Part print with two shaded views. Sizes in mm from the minimum x, y, z corner. A direction names the side the tool comes from. Round coordinates to 2 decimals unless told otherwise and drop trailing zeros. Loops run counter-clockwise (first coordinate to the right, second up) from the corner with the lowest first, then second, coordinate; pieces in that order, holes last. Notation, with made-up numbers: (66.5, 36.5) - (95.5, 36.5) arc R29 ccw to (95.5, 57.5) - close; hole circle Ø7 at (19, -8.5). An arc over 180 degrees is marked (long way). One line per question, with ' | ' between items.
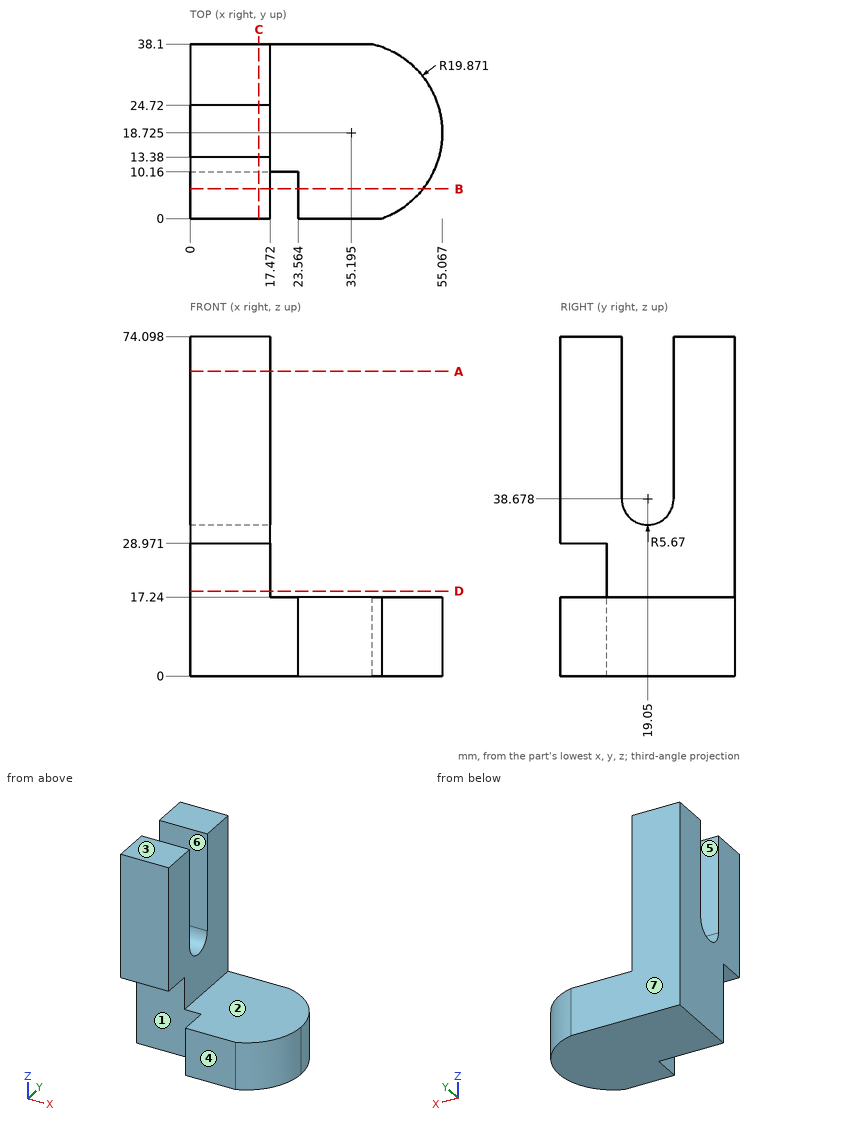
(1) Two-plate mould, pull along Y, no slides. Class the marked faces 4, 5, 6 and 7: released by +Y, released by -Y, zero draft, split by the parting line, or undercut.
Results found:
face 4: released by -Y | face 5: undercut | face 6: undercut | face 7: released by +Y
(2) Probe L1, parallel to Z at x = 34, y = 27; L2, parallel to X at y = 22, z = 22.5; L3, parallel to Y at x = 14.5, z = 18. List the from-to ranges inside material, lowest first.
Results found:
L1: z = 0 to 17.24 | L2: x = 0 to 17.47 | L3: y = 10.16 to 38.1
(3) Cut at A-A, the plane z = 66.5. Write the cut outline in (x, y).
Results found:
outline: (0, 0) - (17.47, 0) - (17.47, 13.38) - (0, 13.38) - close; (0, 24.72) - (17.47, 24.72) - (17.47, 38.1) - (0, 38.1) - close
(4) Cut at D-D, the plane z = 18.5. Write the cut outline in (x, y).
Results found:
outline: (0, 10.16) - (17.47, 10.16) - (17.47, 38.1) - (0, 38.1) - close
(5) Cut at B-B, the plane y = 6.5. Write the cut outline in (x, z) (1 decimal), then the cut area to 3 significant figures.
Results found:
outline: (0, 29) - (17.5, 29) - (17.5, 74.1) - (0, 74.1) - close; (23.6, 0) - (50.9, 0) - (50.9, 17.2) - (23.6, 17.2) - close | area: 1,260 mm²
(6) Drop flat-ended pins along their axis: P1, Ø5, axis at x = 6, y = 3.5, coming from the -Z side; P2, Ø12, axis at y = 34, z = 29.5, coming from the +X side; P3, Ø19, axis at x = 11, z = 15, coming from the -Y side. Give the stop position or say it passes through.
Results found:
P1: stops at z = 28.97 | P2: stops at x = 17.47 | P3: stops at y = 10.16
(7) Cut at C-C, the plane x = 15. Write the cut outline in (y, z), then the cut area to 3 significant figures.
Results found:
outline: (0, 28.97) - (10.16, 28.97) - (10.16, 0) - (38.1, 0) - (38.1, 74.1) - (24.72, 74.1) - (24.72, 38.68) arc R5.67 cw to (13.38, 38.68) - (13.38, 74.1) - (0, 74.1) - close | area: 2,080 mm²
(8) Tool access for the marked faces 1, 2 and 3: list every direction of +Z, -Z, +X, -X, +Y, -Y with a clear straight run to the whole face (end or side of a thin tool).
Results found:
face 1: -Z, -X, -Y | face 2: +Z, +X, +Y, -Y | face 3: +Z, +X, -X, +Y, -Y
